Autodesk Inventor part; units mm, degrees
ref_plane "YZ Plane" through (0, 0, 0) normal (1, 0, 0) x (0, 1, 0)
ref_plane "XZ Plane" through (0, 0, 0) normal (0, 1, 0) x (-1, 0, 0)
ref_plane "XY Plane" through (0, 0, 0) normal (0, 0, 1) x (1, 0, 0)
sketch "Sketch1" plane through (0, 0, 0) normal (0, 1, 0) x (-1, 0, 0)
  line L0 (-90, -90) -> (90, -90)
  line L1 (90, -90) -> (90, 90)
  line L2 (90, 90) -> (-90, 90)
  line L3 (-90, 90) -> (-90, -90)
  line L4 (-90, -90) -> (90, 90) construction
  line L5 (90, -90) -> (-90, 90) construction
  point P0 (0, 0)
  dimension "d0" = 180
  dimension "d1" = 180
extrude "Extrusion1" add sketch "Sketch1" along normal blind 6.35
sketch "Sketch2" plane through (0, 6.35, 0) normal (0, 1, 0) x (1, 0, 0)
  point P0 (0, 0)
  point P1 (-80, -80)
  point P2 (-80, 80)
  point P3 (80, 80)
  point P4 (80, -80)
  dimension "d4" = 160
  dimension "d5" = 80
  dimension "d6" = 160
  dimension "d7" = 80
hole "Hole1" at (-80, 6.35, 80) at (-80, 6.35, -80) at (80, 6.35, -80) at (80, 6.35, 80) direction (0, -1, 0) diameter 5.5 end through all countersink diameter 10.4 countersink angle 90
sketch "Sketch3" plane through (0, 6.35, 0) normal (0, 1, 0) x (1, 0, 0)
  point P0 (0, 0)
  point P1 (-25.4, 76.2)
  point P2 (-25.4, -76.2)
  point P3 (25.4, -76.2)
  point P4 (25.4, 76.2)
  point P5 (0, -76.2)
  point P6 (0, 76.2)
  point P7 (-50.8, 76.2)
  point P8 (-50.8, -76.2)
  point P9 (50.8, -76.2)
  point P10 (50.8, 76.2)
  dimension "d15" = 152.4
  dimension "d16" = 50.8
  dimension "d17" = 76.2
  dimension "d18" = 25.4
  dimension "d27" = 25.4
  dimension "d28" = 25.4
hole "Hole2" at (-25.4, 6.35, -76.2) at (-25.4, 6.35, 76.2) at (25.4, 6.35, 76.2) at (25.4, 6.35, -76.2) at (0, 6.35, 76.2) at (-50.8, 6.35, 76.2) at (50.8, 6.35, 76.2) at (50.8, 6.35, -76.2) at (0, 6.35, -76.2) at (-50.8, 6.35, -76.2) direction (0, -1, 0) diameter 4.9784 end through all
fillet "Fillet1" radius 5 4 edges at (90, 3.175, 90) (90, 3.175, -90) (-90, 3.175, -90) (-90, 3.175, 90)
properties part number "Chuck Adapter Plate"
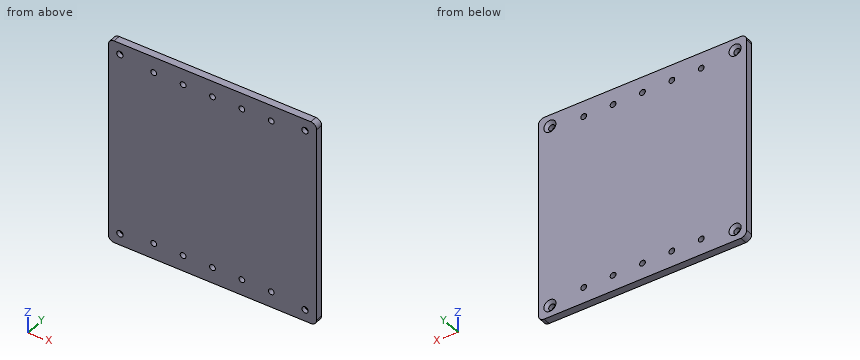
Verification items for the finished model (mm, model axes). Give positions to 0.01 mm unless a question says otherwise; leave off trailing zeros. Order: outer loops, then holes, each group sorted by start corner. A loop starts at its lowest first (then second) coordinate and runs counter-clockwise, first axis right, second up. Notation, with made-up numbers: (84.5, 1.25) - (127.5, 1.25) arc R25 cw to (127.5, 29.25) - close; hole circle Ø6 at (16, -24). An arc over 180 degrees is marked (long way). Answer as CSV lines item,"result". Start each with the question number.
Item 1: Gauge pin test, flat end, axial feed: pin 1 (3 mm diameter, centred on x = 50.8, z = 76.2, fed in from -Y). Record the tip position at first contact, or that the pin passes through.
Item 2: Section check A-A, the plane x = -80. Record the boundary of the cut face in (y, z), plus the area to 3 significant figures.
Item 3: Material ranges on L1, parallel to Z at x = -80, y = 1.7; L2, parallel to X at y = 2.5, z = 76.2, recorded low to high.
Item 4: Section check B-B, the plane x = -50.8. Record the boundary of the cut face in (y, z), plus the area to 3 significant figures.
Filled in:
1,pin 1,"through"
2,outline,"(0, -90) - (6.35, -90) - (6.35, -85.2) - (3.9, -82.75) - (0, -82.75) - close; (0, -77.25) - (3.9, -77.25) - (6.35, -74.8) - (6.35, 74.8) - (3.9, 77.25) - (0, 77.25) - close; (0, 82.75) - (3.9, 82.75) - (6.35, 85.2) - (6.35, 90) - (0, 90) - close"
2,area,"1,060 mm^2"
3,L1,"-90 to -82.75, -77.25 to 77.25, 82.75 to 90"
3,L2,"-90 to -53.29, -48.31 to -27.89, -22.91 to -2.49, 2.49 to 22.91, 27.89 to 48.31, 53.29 to 90"
4,outline,"(0, -90) - (6.35, -90) - (6.35, -78.69) - (0, -78.69) - close; (0, -73.71) - (6.35, -73.71) - (6.35, 73.71) - (0, 73.71) - close; (0, 78.69) - (6.35, 78.69) - (6.35, 90) - (0, 90) - close"
4,area,"1,080 mm^2"
